Verification items for the finished model (mm, model axes). Face numbers are marked on the shaded views. A direction names the side the tool comes from. Coordinates: 2 decimals unless noted, no trailing zeros. Order: outer loops, then holes, each group sorted by start corner. A loop starts at its lowest first (then second) coordinate and runs counter-clockwise, first axis right, second up. Notation, with made-up numbers: M 47.25,-20 L 94.25,-20 A18 ccw 94.25,7 Z; hole C 82.5,76.5 d11. An arc over 180 degrees is marked long. Return JSON: item names as keys, results as strings.
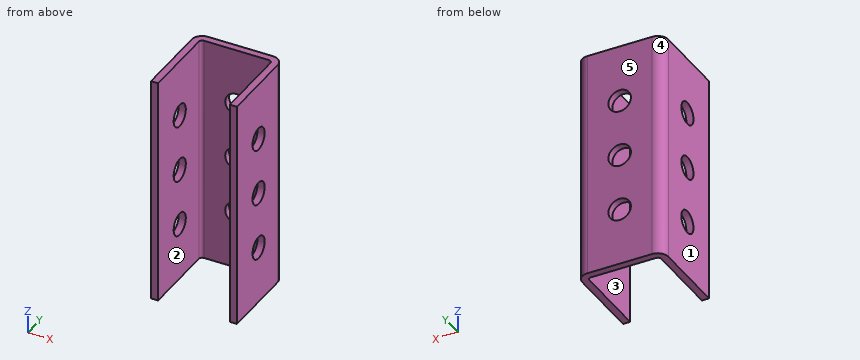
```python
from build123d import *

# Parameters (mm, degrees)
BASE_FLANGE1_DEPTH = 50.8
SKETCH6_R          = 2.4892
CUT_EXTRUDE1_DEPTH = 56.084191244
SKETCH7_R          = 2.4892
CUT_EXTRUDE2_DEPTH = 58.501695627


# Sheet-metal steps are written as plain solids
with BuildPart() as part:
    # Sketch1 → Base-Flange1 (new body)
    with BuildSketch(Plane.XY):
        with BuildLine():
            Line((-9.525, 0), (-9.525, 16.7005))
            ThreePointArc((-9.525, 16.7005), (-8.836847382, 18.361847382), (-7.1755, 19.05))
            Line((-7.1755, 19.05), (7.1755, 19.05))
            ThreePointArc((7.1755, 19.05), (8.836847382, 18.361847382), (9.525, 16.7005))
            Line((9.525, 16.7005), (9.525, 0))
            Line((9.525, 0), (7.9375, 0))
            Line((7.9375, 0), (7.9375, 16.7005))
            ThreePointArc((7.9375, 16.7005), (7.714315367, 17.239315367), (7.1755, 17.4625))
            Line((7.1755, 17.4625), (-7.1755, 17.4625))
            ThreePointArc((-7.1755, 17.4625), (-7.714315367, 17.239315367), (-7.9375, 16.7005))
            Line((-7.9375, 16.7005), (-7.9375, 0))
            Line((-7.9375, 0), (-9.525, 0))
        make_face()
    extrude(amount=BASE_FLANGE1_DEPTH)

    # Sketch6 → Cut-Extrude1 (cut, through all)
    with BuildSketch(Plane(origin=(0, 19.05, 0), x_dir=(1, 0, 0), z_dir=(0, 1, 0))):
        with Locations(Location((0, -12.7, 0), (0, 0, 270))):
            Circle(SKETCH6_R)
        with Locations(Location((0, -25.4, 0), (0, 0, 270))):
            Circle(SKETCH6_R)
        with Locations(Location((0, -38.1, 0), (0, 0, 270))):
            Circle(SKETCH6_R)
    extrude(amount=-CUT_EXTRUDE1_DEPTH, mode=Mode.SUBTRACT)

    # Sketch7 → Cut-Extrude2 (cut, through all)
    with BuildSketch(Plane(origin=(9.525, 0, 0), x_dir=(0, 0, -1), z_dir=(1, 0, 0))):
        with Locations((-25.4, 8.89)):
            Circle(SKETCH7_R)
        with Locations((-12.7, 8.89)):
            Circle(SKETCH7_R)
        with Locations((-38.1, 8.89)):
            Circle(SKETCH7_R)
    extrude(amount=-CUT_EXTRUDE2_DEPTH, mode=Mode.SUBTRACT)


solid = part.part
```
Q1. Material ranges on line 1 along X through (y, z) = (13, 9.5) (1 decimal); line 2 along Y through (x, z) = (-3, 26); line 3 along Y through (x, z) = (8.95, 38.1), recorded low to high.
Values:
{"line 1": "-9.5 to -7.9, 7.9 to 9.5", "line 2": "17.46 to 19.05", "line 3": "0 to 6.4, 11.38 to 18.24"}
Q2. Cross-section at B-B, the plane y = 15.25. Record the boundary of the cut face in (x, z) (1 decimal).
Values:
{"outline": "M -9.5,0 L -7.9,0 L -7.9,50.8 L -9.5,50.8 Z; M 7.9,0 L 9.5,0 L 9.5,50.8 L 7.9,50.8 Z"}
Q3. Tool access check on the marked faces 1 and 2. Record the directions out of +Z, -Z, +X, -X, +Y, -Y that give a thin tool (end or side, any length) a straight path to the whole face; none if there is none.
Values:
{"face 1": "+Z, -Z, -X, +Y, -Y", "face 2": "+Z, -Z, -Y"}
Q4. Go/stop test with flat-tipped pins: pin 1 (3 mm diameter, centred on x = 0, z = 38.1, fed in from -Y); pin 2 (1 mm diameter, centred on x = 7.5, z = 7, fed in from +Y); pin 3 (5.5 mm diameter, centred on x = 0, z = 12.7, fed in from -Y). Record where each tip stops, or that it passes through.
Values:
{"pin 1": "through", "pin 2": "y = 19.05", "pin 3": "y = 17.46"}
Q5. Draft check along X on the marked faces 3, 4 and 5. Enter one of: pulls with the +X half, pulls with the -X half, needs draft (parallel to the pull), parting line crosses it, or undercut.
Values:
{"face 3": "undercut", "face 4": "pulls with the -X half", "face 5": "needs draft"}
Q6. Cross-section at A-A, the plane z = 38.1. State how many separate pieces and enclosed holes the cut face has, and give its area (3 significant figures).
Values:
{"separate pieces": "4", "enclosed holes": "0", "area": "59.9 mm^2"}
